Part model, mm, in its own coordinate system. A direction names the side the tool comes from. Give positions to 0.01 mm unless a question says otherwise; leave off trailing zeros. Order: outer loops, then holes, each group sorted by start corner. A loop starts at its lowest first (then second) coordinate and runs counter-clockwise, first axis right, second up.
1. Slice it at B-B on z = 0.4. List the corners of the cut face in (x, y), and give its area (3 significant figures).
2. Which spindle directions (+Z, -Z, +X, -X, +Y, -Y) get a long thin tool onto all of the face, cutting with end or side? Do faces 5 (the cylindrical face through (0, 5.51, -0.07)), 6 (the flat face through (3.099, 0, 0)). Say none if no direction does.
3. Slice it at D-D on z = 1.2. List the corners of the cut face in (x, y), and give its area (3 significant figures).
4. Mould opens along X. For faces 1 (the flat face through (0.305, 0, 0)), 2 (the cylindrical face through (1.721, 4.467, 1.348)), 3 (the flat face through (-0.305, 0, 0)), 4 (the cylindrical face through (0, -5.51, 0.07)) say: +X half, -X half, draft (parallel to the pull), parting line (faces both ways), or undercut.
5. Slice it at C-C on x = 2. List the corners of the cut face in (y, z).
6. Probe line 1 (Y direction, x = 1.25, z = -0.7); line 2 (X direction, y = -1, z = 1.3); line 3 (Y direction, x = 0.4, z = -0.3). List the from-to ranges inside material, lowest first.
7. Slice it at A-A on y = 3. List the corners of the cut face in (x, z), and give its area (3 significant figures).
8. Drop flat-ended pins along their axis: pin 1 Ø2 at (x, y) = (0.5, -2) entering from -Z; pin 2 Ø1.5 at (y, z) = (3, 0) entering from +X; pin 3 Ø0.5 at (x, y) = (3.5, -0.5) entering from -Z. Give the stop position or say it passes through.
from build123d import *

# Parameters (mm, degrees)
F0_R     = 0.9144
F1_DEPTH = 0.3048
F2_R     = 1.9939
F2_R_2   = 0.9144
F3_DEPTH = 1.397
F8_DEPTH = 0.6096


# Not quite as in the source:
# - a pattern or mirror of a feature is missing from the dataset's text; its kind, count and spacing are read off the source's solid


with BuildPart() as f1:
    # F0 (on Right) → F1 (new body, symmetric)
    with BuildSketch(Plane.YZ):
        with BuildLine():
            ThreePointArc((2.1201945262, 2.3567084162), (0, 2.094238318), (-2.1201945262, 2.3567084162))
            ThreePointArc((-2.1201945262, 2.3567084162), (-5.5118, 0), (-2.1201945262, -2.3567084162))
            ThreePointArc((-2.1201945262, -2.3567084162), (0, -2.094238318), (2.1201945262, -2.3567084162))
            ThreePointArc((2.1201945262, -2.3567084162), (5.5118, 0), (2.1201945262, 2.3567084162))
        make_face()
        with Locations((-2.9972, 0)):
            Circle(F0_R, mode=Mode.SUBTRACT)
        with Locations((2.9972, 0)):
            Circle(F0_R, mode=Mode.SUBTRACT)
    extrude(amount=F1_DEPTH, both=True)

    # F2 (on face) → F3 (join)
    with BuildSketch(Plane.YZ.offset(0.3048)):
        with Locations((-2.9972, 0)):
            Circle(F2_R)
        with Locations((-2.9972, 0)):
            Circle(F2_R_2, mode=Mode.SUBTRACT)
    extrude(amount=F3_DEPTH)

    # F4: F1 across plane


with BuildPart() as f1_1:
    add(f1.part)
    add(f1.part.mirror(Plane.XZ))

    # F5: F1 across face


with BuildPart() as f1_2:
    add(f1_1.part)
    add(f1_1.part.mirror(Plane(origin=(1.7018, -2.9972, 0), x_dir=(0, 1, 0), z_dir=(1, 0, 0))))

    # F7 (on face) → F8 (join, through all)
    with BuildSketch(Plane.YZ.offset(3.7084)):
        Polygon((1.7045348049, -2.2), (0, 0), (-1.6570564457, -2.2), align=None)
    f8 = extrude(amount=-F8_DEPTH)

    # F8_copies: F8 across plane
    add(f8.mirror(Plane.XY))


solid = f1_2.part
Data:
1. outline: (-0.3, -5.48) - (0.3, -5.48) - (0.3, -4.95) - (3.1, -4.95) - (3.1, -5.48) - (3.71, -5.48) - (3.71, -3.82) - (-0.3, -3.82) - close; (-0.3, -2.17) - (3.71, -2.17) - (3.71, 2.17) - (-0.3, 2.17) - close; (-0.3, 3.82) - (3.71, 3.82) - (3.71, 5.48) - (3.1, 5.48) - (3.1, 4.95) - (0.3, 4.95) - (0.3, 5.48) - (-0.3, 5.48) - close; hole (0.3, -1.04) - (3.1, -1.04) - (3.1, 1.04) - (0.3, 1.04) - close
1. area: 22.0 mm2
2. face 5: +X, -X
2. face 6: none
3. outline: (-0.3, -5.21) - (0.3, -5.21) - (0.3, -4.59) - (3.1, -4.59) - (3.1, -5.21) - (3.71, -5.21) - (3.71, 5.21) - (3.1, 5.21) - (3.1, 4.59) - (0.3, 4.59) - (0.3, 5.21) - (-0.3, 5.21) - close; hole (0.3, -1.4) - (3.1, -1.4) - (3.1, 1.4) - (0.3, 1.4) - close
3. area: 30.5 mm2
4. face 1: undercut
4. face 2: undercut
4. face 3: -X half
4. face 4: draft
5. outline: circle Ø3.99 at (-3, 0); circle Ø3.99 at (3, 0); hole circle Ø1.83 at (-3, 0); hole circle Ø1.83 at (3, 0)
6. line 1: y = -4.86 to -3.59, -2.41 to -1.13, 1.13 to 2.41, 3.59 to 4.86
6. line 2: x = -0.3 to 0.3, 3.1 to 3.71
6. line 3: y = -4.97 to -3.86, -2.13 to -1.03, 1.03 to 2.13, 3.86 to 4.97
7. outline: (-0.3, -2.51) - (0.3, -2.51) - (0.3, -1.99) - (3.1, -1.99) - (3.1, -2.51) - (3.71, -2.51) - (3.71, -0.91) - (-0.3, -0.91) - close; (-0.3, 0.91) - (3.71, 0.91) - (3.71, 2.51) - (3.1, 2.51) - (3.1, 1.99) - (0.3, 1.99) - (0.3, 2.51) - (-0.3, 2.51) - close
7. area: 9.93 mm2
8. pin 1: stops at z = -2.51
8. pin 2: passes through
8. pin 3: stops at z = -2.2
